Source: CAD feature listing. Evaluate the final solid. Frame: model axes, mm. A direction names the side the tool comes from. Coordinates: 2 decimals unless noted, no trailing zeros. Loops run counter-clockwise (first coordinate to the right, second up) from the corner with the lowest first, then second, coordinate; pieces in that order, holes last. Notation, with made-up numbers: (21.5, 32.5) - (26.5, 32.5) arc R25 cw to (26.5, 44.5) - close; hole circle Ø5 at (-3, -22). An arc over 180 degrees is marked (long way). Write item = value, one per line. Start each with the question number.
from build123d import *

# Parameters (mm, degrees)
AUFSATZ_LINEAR_AUSTRAGEN1_DEPTH                = 12
SKIZZE4_R                                      = 4.7
SCHNITT_LINEAR_AUSTRAGEN1_DEPTH                = 8.5
STIRNSENKUNG_START                             = 5.6
STIRNSENKUNG_F_R_M3_ZYLINDERSCHRAUBE_2_R       = 3.25
STIRNSENKUNG_F_R_M3_ZYLINDERSCHRAUBE_MIT_DEPTH = 3.4
STIRNSENKUNG_START_2                           = 14.1
STIRNSENKUNG_F_R_M3_ZYLINDERSCHRAUBE_3_O_R     = 3.25
STIRNSENKUNG_F_R_M3_ZYLINDERSCHRAUBE_3_DEPTH   = 3.4
STIRNSENKUNG_F_R_M3_ZYLINDERSCHRAUBE_4_O_R     = 1.6
STIRNSENKUNG_F_R_M3_ZYLINDERSCHRAUBE_4_DEPTH   = 5.6
STIRNSENKUNG_START_3                           = 11
STIRNSENKUNG_F_R_M3_ZYLINDERSCHRAUBE_5_O_R     = 1.6
STIRNSENKUNG_F_R_M3_ZYLINDERSCHRAUBE_5_DEPTH   = 3.1


# Read off the part's stored shape, not the designer's step: Stirnsenkung für M3 Zylinderschraube mit Innensechskant1
with BuildPart() as part:
    # Skizze1 → Aufsatz-Linear austragen1 (new body)
    with BuildSketch(Plane.XY):
        with BuildLine():
            Line((0, 0), (54, 0))
            Line((54, 0), (54, 9))
            Line((54, 9), (34.5, 9))
            Line((34.5, 9), (34.5, 17.5))
            Line((34.5, 17.5), (12, 17.5))
            Line((12, 17.5), (12, 11))
            Line((12, 11), (22.998047352, 11))
            ThreePointArc((22.998047352, 11), (31.125, 10), (22.998047352, 9))
            Line((22.998047352, 9), (0, 9))
            Line((0, 9), (0, 0))
        make_face()
    extrude(amount=AUFSATZ_LINEAR_AUSTRAGEN1_DEPTH)

    # Skizze4 → Schnitt-Linear austragen1 (cut)
    with BuildSketch(Plane.XY.offset(12)):
        with Locations((27, 10)):
            Circle(SKIZZE4_R)
    extrude(amount=-SCHNITT_LINEAR_AUSTRAGEN1_DEPTH, mode=Mode.SUBTRACT)

    # Stirnsenkung f_r M3 Zylinderschraube 2 → Stirnsenkung für M3 Zylinderschraube mit Innensechskant1 (cut)
    with BuildSketch(Plane(origin=(0, 0, 0), x_dir=(1, 0, 0), z_dir=(0, 1, 0)).offset(STIRNSENKUNG_START)):
        with Locations((48, -6)):
            Circle(STIRNSENKUNG_F_R_M3_ZYLINDERSCHRAUBE_2_R)
        with Locations((6, -6)):
            Circle(STIRNSENKUNG_F_R_M3_ZYLINDERSCHRAUBE_2_R)
    extrude(amount=STIRNSENKUNG_F_R_M3_ZYLINDERSCHRAUBE_MIT_DEPTH, mode=Mode.SUBTRACT)

    # Stirnsenkung f_r M3 Zylinderschraube 3 o → Stirnsenkung f_r M3 Zylinderschraube 3 (cut)
    with BuildSketch(Plane(origin=(0, 0, 0), x_dir=(1, 0, 0), z_dir=(0, 1, 0)).offset(STIRNSENKUNG_START_2)):
        with Locations((18, -6)):
            Circle(STIRNSENKUNG_F_R_M3_ZYLINDERSCHRAUBE_3_O_R)
    extrude(amount=STIRNSENKUNG_F_R_M3_ZYLINDERSCHRAUBE_3_DEPTH, mode=Mode.SUBTRACT)

    # Stirnsenkung f_r M3 Zylinderschraube 4 o → Stirnsenkung f_r M3 Zylinderschraube 4 (cut)
    with BuildSketch(Plane(origin=(0, 0, 0), x_dir=(1, 0, 0), z_dir=(0, 1, 0))):
        with Locations((48, -6)):
            Circle(STIRNSENKUNG_F_R_M3_ZYLINDERSCHRAUBE_4_O_R)
        with Locations((6, -6)):
            Circle(STIRNSENKUNG_F_R_M3_ZYLINDERSCHRAUBE_4_O_R)
    extrude(amount=STIRNSENKUNG_F_R_M3_ZYLINDERSCHRAUBE_4_DEPTH, mode=Mode.SUBTRACT)

    # Stirnsenkung f_r M3 Zylinderschraube 5 o → Stirnsenkung f_r M3 Zylinderschraube 5 (cut)
    with BuildSketch(Plane(origin=(0, 0, 0), x_dir=(1, 0, 0), z_dir=(0, 1, 0)).offset(STIRNSENKUNG_START_3)):
        with Locations((18, -6)):
            Circle(STIRNSENKUNG_F_R_M3_ZYLINDERSCHRAUBE_5_O_R)
    extrude(amount=STIRNSENKUNG_F_R_M3_ZYLINDERSCHRAUBE_5_DEPTH, mode=Mode.SUBTRACT)


solid = part.part
Item 1: Cut plane A-A (z = 6). State how many separate pieces and enclosed holes the cut face has, then the cut area to 3 significant figures.
Item 2: First-contact query: pin 1 (4 mm diameter, centred on x = 48, z = 6, fed in from +Y); pin 2 (7 mm diameter, centred on y = 14, z = 8, fed in from -X); pin 3 (5 mm diameter, centred on x = 5, z = 7, fed in from +Y). Flat tips, straight axial feed; report the tip coordinate or a pass-through.
Item 3: Cut plane B-B (x = 48). Return the cut outline in (y, z), then the cut area to 3 significant figures.
Item 4: Draft query along Y for faces 4 (the flat face through (7.4, 5.6, 7.4)), 5 (the cylindrical face through (16.73, 12.53, 6.97)), 6 (the flat face through (16, 11, 6)). Return one class per face: released by +Y, released by -Y, zero draft, split by the parting line, or undercut.
Item 5: Cut plane C-C (x = 18). Return the cut outline in (y, z), then the cut area to 3 significant figures.
Item 6: Material intervals for L1, parallel to X at y = 2.05, z = 6; L2, parallel to Z at x = 48, y = 2; L3, parallel to X at y = 7.5, z = 8, sorted ascending. Write a range as [from, to].
Item 7: Cut plane D-D (y = 10). Return the cut outline in (x, z) (3 decimals).
Item 8: Reachability of faces 1 (the cylindrical face through (31.696, 9.807, 7.81)), 2 (the flat face through (12, 14, 6)), 3 (the cylindrical face through (7.5, 7.276, 8.883)) from +Z, -Z, +X, -X, +Y, -Y: full face, straight path, thin tool, end or side. Return the list, or none.
Responses:
q1.separate_pieces = 4
q1.enclosed_holes = 0
q1.area = 475 mm2
q2.pin_1 = 5.6
q2.pin_2 = 12
q2.pin_3 = 9
q3.outline = (0, 0) - (9, 0) - (9, 2.75) - (5.6, 2.75) - (5.6, 4.4) - (0, 4.4) - close; (0, 7.6) - (5.6, 7.6) - (5.6, 9.25) - (9, 9.25) - (9, 12) - (0, 12) - close
q3.area = 68.0 mm2
q4.face_4 = released by +Y
q4.face_5 = zero draft
q4.face_6 = undercut
q5.outline = (0, 0) - (9, 0) - (9, 12) - (0, 12) - close; (11, 0) - (17.5, 0) - (17.5, 2.75) - (14.1, 2.75) - (14.1, 4.4) - (11, 4.4) - close; (11, 7.6) - (14.1, 7.6) - (14.1, 9.25) - (17.5, 9.25) - (17.5, 12) - (11, 12) - close
q5.area = 154 mm2
q6.L1 = [0, 4.4], [7.6, 46.4], [49.6, 54]
q6.L2 = [0, 4.4], [7.6, 12]
q6.L3 = [0, 3.44], [8.56, 23.02], [30.98, 45.44], [50.56, 54]
q7.outline = (31.125, 0) - (34.5, 0) - (34.5, 12) - (31.7, 12) - (31.7, 3.5) - (31.125, 3.5) - close
q8.face_1 = +Z
q8.face_2 = +Z, -Z, -X, +Y
q8.face_3 = +Y
